```python
from build123d import *

# Parameters (mm, degrees)
ESBO_O1_R                  = 20.588327932
RESSALTO_EXTRUS_O1_DEPTH   = 70
ESBO_O2_R                  = 28.781927243
RESSALTO_EXTRUS_O2_DEPTH   = 10
ESBO_O4_R                  = 28.78
RESSALTO_EXTRUS_O3_DEPTH   = 10
ESBO_O5_R                  = 19
CORTE_EXTRUS_O4_DEPTH      = 90
CORTE_EXTRUS_O5_DEPTH      = 90.759671744
CORTE_EXTRUS_O5_DEPTH_BACK = 90.759671744
CORTE_EXTRUS_O6_DEPTH      = 90.759671833
CORTE_EXTRUS_O6_DEPTH_BACK = 90.759671833


with BuildPart() as part:
    # Esboço1 → Ressalto-extrusão1 (new body)
    with BuildSketch(Plane(origin=(0, 0, 0), x_dir=(1, 0, 0), z_dir=(0, 1, 0))):
        with Locations(Location((0, 0, 0), (0, 0, 270))):
            Circle(ESBO_O1_R)
    extrude(amount=RESSALTO_EXTRUS_O1_DEPTH)

    # Esboço2 → Ressalto-extrusão2 (add)
    with BuildSketch(Plane.XZ):
        with Locations(Location((0, 0, 0), (0, 0, 270))):
            Circle(ESBO_O2_R)
    extrude(amount=RESSALTO_EXTRUS_O2_DEPTH)

    # Esboço4 → Ressalto-extrusão3 (add)
    with BuildSketch(Plane(origin=(0, 70, 0), x_dir=(1, 0, 0), z_dir=(0, 1, 0))):
        with Locations(Location((0, 0, 0), (0, 0, 270))):
            Circle(ESBO_O4_R)
    extrude(amount=RESSALTO_EXTRUS_O3_DEPTH)

    # Esboço5 → Corte-extrusão4 (cut)
    with BuildSketch(Plane(origin=(0, 80, 0), x_dir=(1, 0, 0), z_dir=(0, 1, 0))):
        with Locations(Location((0, 0, 0), (0, 0, 270))):
            Circle(ESBO_O5_R)
    extrude(amount=-CORTE_EXTRUS_O4_DEPTH, mode=Mode.SUBTRACT)

    # Esboço6 → Corte-extrusão5 (cut, two sides: drawn at the far end of the back side and taken through both)
    with BuildSketch(Plane(origin=(0, 0, 0), x_dir=(0, 0, -1), z_dir=(1, 0, 0)).offset(-CORTE_EXTRUS_O5_DEPTH_BACK)):
        with BuildLine():
            Line((6.956334081, 55.558451616), (6.956334081, 17.919715425))
            ThreePointArc((6.956334081, 17.919715425), (0, 10.963381344), (-6.956334081, 17.919715425))
            Line((-6.956334081, 17.919715425), (-6.956334081, 55.558451616))
            ThreePointArc((-6.956334081, 55.558451616), (0, 62.514785697), (6.956334081, 55.558451616))
        make_face()
    extrude(amount=CORTE_EXTRUS_O5_DEPTH + CORTE_EXTRUS_O5_DEPTH_BACK, mode=Mode.SUBTRACT)

    # Esboço7 → Corte-extrusão6 (cut, two sides: drawn at the far end of the back side and taken through both)
    with BuildSketch(Plane.XY.offset(-CORTE_EXTRUS_O6_DEPTH_BACK)):
        with BuildLine():
            Line((6.707893579, 57.67019589), (6.707893579, 15.062649642))
            ThreePointArc((6.707893579, 15.062649642), (0, 8.354756063), (-6.707893579, 15.062649642))
            Line((-6.707893579, 15.062649642), (-6.707893579, 57.67019589))
            ThreePointArc((-6.707893579, 57.67019589), (0, 64.378089469), (6.707893579, 57.67019589))
        make_face()
    extrude(amount=CORTE_EXTRUS_O6_DEPTH + CORTE_EXTRUS_O6_DEPTH_BACK, mode=Mode.SUBTRACT)


solid = part.part
```
Check sheet for the modelled part. Datum: model origin and axes. Units: mm. A direction names the side the tool comes from. Round coordinates to 2 decimals unless told otherwise and drop trailing zeros. Loops run counter-clockwise (first coordinate to the right, second up) from the corner with the lowest first, then second, coordinate; pieces in that order, holes last. Notation, with made-up numbers: (-14, 7.25) - (26, 7.25) arc R29 ccw to (26, 34.25) - close; hole circle Ø1 at (15.25, 53.5). An arc over 180 degrees is marked (long way). Write item = value, one per line. Start each with the question number.
Q1. Access from +Z, -Z, +X, -X, +Y, -Y to the whole of each face (thin tool, end or side, straight path). Record for faces 4 (the face through (19.442, 62.513, 0.153)), 5 (the face through (20, 0, 7)), 6 (the face through (0.148, 8.356, 19.163)).
Q2. Depth check by flat-ended pin: P1, Ø0.8, axis at y = 44.5, z = 18.5, coming from the +X side; P2, Ø2, axis at y = 12, z = 9.5, coming from the +X side; P3, Ø1.4, axis at y = 42, z = 18.5, coming from the -X side. Enter the tip coordinate at first touch or a pass-through.
Q3. Section check A-A (y = 19.5). Record the boundary of the cut face in (x, z), plus the area to 3 significant figures.
Q4. Section check B-B (z = 0). Record the boundary of the cut face in (x, y), plus the area to 3 significant figures.
Q5. Thickness scan on L1, parallel to X at y = 8, z = 0; L2, parallel to Y at x = 21, z = -14; L3, parallel to Z at x = -13, y = 55.5. Record the ranges inside material, lowest first.
Q6. Section check C-C (x = 0). Record the boundary of the cut face in (y, z), plus the area to 3 significant figures.
Q7. Release check for a two-part mould opening along Z. For faces 1 (the face through (-16.856, 35.63, 8.767)), 2 (the face through (20, 70, -7)), 3 (the face through (-7.885, 34.51, 19.018)) record: pulls with the +Z half, pulls with the -Z half, needs draft (parallel to the pull), parting line crosses it, or undercut.
Q8. Section check D-D (z = 9.5). Record the boundary of the cut face in (x, y), plus the area to 3 significant figures.
Derived:
q1.face_4 = +X, -X
q1.face_5 = none
q1.face_6 = +Z, -Z
q2.P1 = 9.81
q2.P2 = 18.75
q2.P3 = -10.35
q3.outline = (-19.38, -6.96) arc R20.59 ccw to (-6.71, -19.46) - (-6.71, -17.78) arc R19 cw to (-17.68, -6.96) - close; (-19.38, 6.96) - (-17.68, 6.96) arc R19 cw to (-6.71, 17.78) - (-6.71, 19.46) arc R20.59 ccw to start; (6.71, -19.46) arc R20.59 ccw to (19.38, -6.96) - (17.68, -6.96) arc R19 cw to (6.71, -17.78) - close; (6.71, 17.78) arc R19 cw to (17.68, 6.96) - (19.38, 6.96) arc R20.59 ccw to (6.71, 19.46) - close
q3.area = 109 mm^2
q4.outline = (-28.78, -10) - (-19, -10) - (-19, 10.96) - (-20.59, 10.96) - (-20.59, 0) - (-28.78, 0) - close; (-28.78, 70) - (-20.59, 70) - (-20.59, 62.51) - (-19, 62.51) - (-19, 80) - (-28.78, 80) - close; (19, -10) - (28.78, -10) - (28.78, 0) - (20.59, 0) - (20.59, 10.96) - (19, 10.96) - close; (19, 62.51) - (20.59, 62.51) - (20.59, 70) - (28.78, 70) - (28.78, 80) - (19, 80) - close
q4.area = 450 mm^2
q5.L1 = -20.59 to -19, 19 to 20.59
q5.L2 = -10 to 0, 70 to 80
q5.L3 = -15.96 to -13.86, 13.86 to 15.96
q6.outline = (-10, -28.78) - (0, -28.78) - (0, -20.59) - (8.35, -20.59) - (8.35, -19) - (-10, -19) - close; (-10, 19) - (8.35, 19) - (8.35, 20.59) - (0, 20.59) - (0, 28.78) - (-10, 28.78) - close; (64.38, -20.59) - (70, -20.59) - (70, -28.78) - (80, -28.78) - (80, -19) - (64.38, -19) - close; (64.38, 19) - (80, 19) - (80, 28.78) - (70, 28.78) - (70, 20.59) - (64.38, 20.59) - close
q6.area = 436 mm^2
q7.face_1 = undercut
q7.face_2 = needs draft
q7.face_3 = parting line crosses it
q8.outline = (-27.17, -10) - (-16.45, -10) - (-16.45, 80) - (-27.17, 80) - (-27.17, 70) - (-18.27, 70) - (-18.27, 0) - (-27.17, 0) - close; (16.45, -10) - (27.17, -10) - (27.17, 0) - (18.27, 0) - (18.27, 70) - (27.17, 70) - (27.17, 80) - (16.45, 80) - close
q8.area = 682 mm^2
